Verification items for the finished model (mm, model axes). Face numbers are marked on the shaded views. Round coordinates to 2 decimals unless told otherwise and drop trailing zeros. Loops run counter-clockwise (first coordinate to the right, second up) from the corner with the lowest first, then second, coordinate; pieces in that order, holes last. Notation, with made-up numbers: M 6,16 L 48,16 A15 cw 48,32 Z; hole C 78.5,41 d2. An arc over 180 degrees is marked long. One line per item, written item: value.
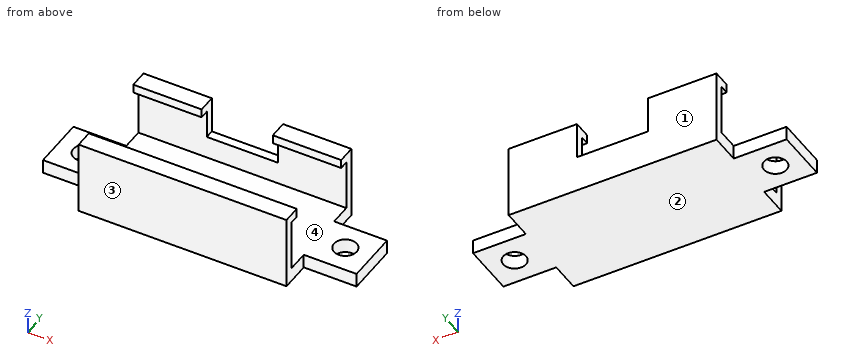
from build123d import *

# Parameters (mm, degrees)
BOSS_EXTRUDE2_DEPTH = 2
SKETCH3_R           = 1.61
CUT_EXTRUDE1_DEPTH  = 7.62
SKETCH6_W           = 29.5
SKETCH6_H           = 1.25
BOSS_EXTRUDE4_DEPTH = 8.5
SKETCH7_W           = 29.5
SKETCH7_H           = 1.25
BOSS_EXTRUDE5_DEPTH = 1.27
SKETCH10_W          = 10.1
SKETCH10_H          = 5.25
CUT_EXTRUDE2_DEPTH  = 2


with BuildPart() as part:
    # Sketch2 → Boss-Extrude2 (new body)
    with BuildSketch(Plane.XY):
        Polygon((0, 4.25), (0, 0), (29.5, 0), (29.5, 4.25), (37, 4.25), (37, 11.75), (29.5, 11.75), (29.5, 16), (0, 16), (0, 11.75), (-7.5, 11.75), (-7.5, 4.25), align=None)
    extrude(amount=-BOSS_EXTRUDE2_DEPTH)

    # Sketch3 → Cut-Extrude1 (cut)
    with BuildSketch(Plane.XY):
        with Locations((33.25, 8)):
            Circle(SKETCH3_R)
        with Locations((-3.75, 8)):
            Circle(SKETCH3_R)
    extrude(amount=-CUT_EXTRUDE1_DEPTH, mode=Mode.SUBTRACT)

    # Sketch6 → Boss-Extrude4 (add)
    with BuildSketch(Plane.XY):
        with Locations((14.75, 0.625)):
            Rectangle(SKETCH6_W, SKETCH6_H)
        with Locations((14.75, 15.375)):
            Rectangle(SKETCH6_W, SKETCH6_H)
    extrude(amount=BOSS_EXTRUDE4_DEPTH)

    # Sketch7 → Boss-Extrude5 (add)
    with BuildSketch(Plane.XZ.offset(-14.75)):
        with Locations((14.75, 7.875)):
            Rectangle(SKETCH7_W, SKETCH7_H)
    boss_extrude5 = extrude(amount=BOSS_EXTRUDE5_DEPTH)

    # Mirror1: Boss-Extrude5 across plane
    add(boss_extrude5.mirror(Plane.ZX.offset(8)))

    # Sketch10 → Cut-Extrude2 (cut, symmetric)
    with BuildSketch(Plane.XZ.offset(-14.75)):
        with Locations((14.75, 5.875)):
            Rectangle(SKETCH10_W, SKETCH10_H)
    extrude(amount=CUT_EXTRUDE2_DEPTH, both=True, mode=Mode.SUBTRACT)


solid = part.part
(1) Sectioned sample at B-B on y = 8. Enter the section's corners in (x, z), and give its area (3 significant figures).
Completed:
outline: M -7.5,-2 L -5.36,-2 L -5.36,0 L -7.5,0 Z; M -2.14,-2 L 31.64,-2 L 31.64,0 L -2.14,0 Z; M 34.86,-2 L 37,-2 L 37,0 L 34.86,0 Z
area: 76.1 mm^2
(2) Mould release check, pull along Y, two halves, no side actions. Record for the marked faces 1, 2, 3 and 4: +Y half, -Y half, draft (parallel to the pull), parting line (faces both ways), or undercut.
Completed:
face 1: +Y half
face 2: draft
face 3: -Y half
face 4: undercut
(3) Sectioned sample at C-C on x = 33.25. Enter the section's corners in (y, z), and give its area (3 significant figures).
Completed:
outline: M 4.25,-2 L 6.39,-2 L 6.39,0 L 4.25,0 Z; M 9.61,-2 L 11.75,-2 L 11.75,0 L 9.61,0 Z
area: 8.56 mm^2
(4) Sectioned sample at D-D on z = 5. Enter the section's corners in (x, y).
Completed:
outline: M 0,0 L 29.5,0 L 29.5,1.25 L 0,1.25 Z; M 0,14.75 L 9.7,14.75 L 9.7,16 L 0,16 Z; M 19.8,14.75 L 29.5,14.75 L 29.5,16 L 19.8,16 Z
(5) Thickness scan on L1, parallel to Y at x = 7, z = 6.5; L2, parallel to Y at x = 33.25, z = -1.55; L3, parallel to X at y = 14, z = -0.75. Record the ranges inside material, lowest first. Write a range as from..to.
Completed:
L1: y = 0..1.25, 14.75..16
L2: y = 4.25..6.39, 9.61..11.75
L3: x = 0..29.5
(6) Sectioned sample at A-A on z = 1. Enter the section's corners in (x, y), and give its area (4 significant figures).
Completed:
outline: M 0,0 L 29.5,0 L 29.5,1.25 L 0,1.25 Z; M 0,14.75 L 29.5,14.75 L 29.5,16 L 0,16 Z
area: 73.75 mm^2
(7) Depth check by flat-ended pin: pin 1 Ø3 at (x, y) = (33.25, 8) entering from -Z; pin 2 Ø4 at (x, y) = (13.5, 9) entering from +Z; pin 3 Ø0.8 at (y, z) = (15, 6) entering from +X; pin 4 Ø3.5 at (y, z) = (14, 4) entering from -X. Enter the tip coordinate at first touch or a pass-through.
Completed:
pin 1: passes through
pin 2: stops at z = 0
pin 3: stops at x = 29.5
pin 4: stops at x = 0
